Check sheet for the modelled part. Datum: model origin and axes. Units: mm. A direction names the side the tool comes from. Coordinates: 2 decimals unless noted, no trailing zeros. Write each loop counter-clockwise with the first axis right and the second up, starting at its lowest first coordinate (ties: lowest second). Pieces come first, ordered by that corner, then holes. Notation, with made-up numbers: (54.25, -33) - (104.25, -33) arc R12 ccw to (104.25, -11) - close; hole circle Ø5 at (66, 64.5). An arc over 180 degrees is marked (long way). Use one line per item in the form item = value. Start each with the question number.
1. Cross-section at A-A on x = 0. Record the boundary of the cut face in (y, z), then the cut area to 3 significant figures.
2. Tool access check on faces 5 (the face through (-10, 0, 138)), 6 (the face through (10.81, -0.07, 131.45)). Record the directions out of +Z, -Z, +X, -X, +Y, -Y that give a thin tool (end or side, any length) a straight path to the whole face; none if there is none.
3. Draft check along X on faces 1 (the face through (0, 0, 0)), 2 (the face through (-15, 0, 74)), 3 (the face through (-1.08, -0.07, 93.12)), 4 (the face through (15, 0, 74)). Enter one of: +X half, -X half, draft (parallel to the pull), parting line (faces both ways), or undercut.
4. Cross-section at C-C on y = 0. Give the number of separate pieces and of enclosed holes in the cut face, then the cut area to 3 significant figures.
5. Cross-section at D-D on x = 10. Record the boundary of the cut face in (y, z).
6. Cross-section at B-B on z = 45. Record the boundary of the cut face in (x, y), then the cut area to 3 significant figures.
7. Scan lines: line 1 along Z through (x, y) = (10, 2.5); line 2 along X through (y, z) = (-0.5, 133); line 3 along X through (y, z) = (1.5, 97.5). Record each from-to range of solid material in increasing order.
8. Go/stop test with a flat-tipped pin: pin 1 Ø1.5 at (x, y) = (10.5, 0) entering from +Z. Record where the tip stops, or that it passes through.
Autodesk Fusion 360 part; units mm, degrees
sketch "Sketch1" plane through (0, 0, 0) normal (0, 0, 1) x (1, 0, 0)
  line L0 (15, 5) -> (-15, 5)
  line L1 (-15, 5) -> (-15, -5)
  line L2 (-15, -5) -> (15, -5)
  line L3 (15, -5) -> (15, 5)
  line L4 (15, 5) -> (-15, -5) construction
  line L5 (-15, 5) -> (15, -5) construction
  dimension "d1" = 30
  dimension "d2" = 10
extrude "Extrude1" add sketch "Sketch1" along normal blind 150
sketch "Sketch2" plane through (0, -5, 0) normal (0, -1, 0) x (1, 0, 0)
  line L0 (-15, 0) -> (15, 0)
  line L1 (15, 0) -> (15, 150)
  line L2 (15, 150) -> (-15, 150)
  line L3 (-15, 150) -> (-15, 0)
  circle A0 centre (0, 118) radius 1.75
  line L4 (0, 150) -> (0, 118)
  circle A1 centre (-10, 133) radius 1.75
  circle A2 centre (10, 133) radius 1.75
  dimension "d5" = 3.5
  dimension "d6" = 32
  dimension "d7" = 3.5
  dimension "d8" = 3.5
  dimension "d9" = 10
  dimension "d10" = 10
  dimension "d11" = 15
  dimension "d12" = 15
extrude "Extrude2" cut sketch "Sketch2" against normal blind 10 contours A0 | A1 | A2
sketch "Sketch3" plane through (0, 0, 150) normal (0, 0, 1) x (-1, 0, 0)
  line L0 (-15, 5) -> (-15, -5)
  line L1 (-15, -5) -> (15, -5)
  line L2 (15, -5) -> (15, 5)
  line L3 (15, 5) -> (-15, 5)
  circle A0 centre (10, 0) radius 2.05
  circle A1 centre (-10, 0) radius 2.05
  dimension "d15" = 4.1
  dimension "d17" = 10
  dimension "d18" = 10
extrude "Extrude3" cut sketch "Sketch3" against normal blind 12 contours A0 | A1
sketch "Sketch4" plane through (0, -5, 0) normal (0, -1, 0) x (1, 0, 0)
  circle A0 centre (-10, 133) radius 1.75
  circle A1 centre (10, 133) radius 1.75
  circle A2 centre (0, 118) radius 1.75
  line L0 (-15, 0) -> (15, 0)
  line L1 (15, 0) -> (15, 150)
  line L2 (15, 150) -> (-15, 150)
  line L3 (-15, 150) -> (-15, 0)
  line L4 (0, 0) -> (0, 6)
  circle A3 centre (0, 15) radius 1.5
  circle A4 centre (-10, 30) radius 1.5
  circle A5 centre (10, 30) radius 1.5
  circle A6 centre (0, 45) radius 1.5
  dimension "d21" = 3
  dimension "d22" = 15
  dimension "d23" = 3
  dimension "d24" = 10
  dimension "d25" = 30
  dimension "d26" = 3
  dimension "d27" = 45
extrude "Extrude4" cut sketch "Sketch4" against normal blind 10 contours A3 | A4 | A5 | A6
sketch "Sketch5" plane through (0, -5, 0) normal (0, -1, 0) x (1, 0, 0)
  circle A0 centre (0, 45) radius 1.5
  circle A1 centre (10, 30) radius 1.5
  circle A2 centre (-10, 30) radius 1.5
  circle A3 centre (0, 15) radius 1.5
  circle A4 centre (-10, 133) radius 1.75
  circle A5 centre (10, 133) radius 1.75
  circle A6 centre (0, 118) radius 1.75
  line L0 (-15, 0) -> (15, 0)
  line L1 (15, 0) -> (15, 150)
  line L2 (15, 150) -> (-15, 150)
  line L3 (-15, 150) -> (-15, 0)
  circle A7 centre (0, 108) radius 1.75
  dimension "d30" = 3.5
  dimension "d31" = 10
extrude "Extrude5" cut sketch "Sketch5" against normal blind 10 contours A7
sketch "Sketch6" plane through (0, -5, 0) normal (0, -1, 0) x (1, 0, 0)
  circle A0 centre (0, 108) radius 1.75
  circle A1 centre (0, 45) radius 1.5
  circle A2 centre (10, 30) radius 1.5
  circle A3 centre (-10, 30) radius 1.5
  circle A4 centre (0, 15) radius 1.5
  circle A5 centre (-10, 133) radius 1.75
  circle A6 centre (10, 133) radius 1.75
  circle A7 centre (0, 118) radius 1.75
  line L0 (-15, 0) -> (15, 0)
  line L1 (15, 0) -> (15, 150)
  line L2 (15, 150) -> (-15, 150)
  line L3 (-15, 150) -> (-15, 0)
  circle A8 centre (0, 98) radius 5
  dimension "d34" = 10
  dimension "d35" = 10
extrude "Extrude6" cut sketch "Sketch6" against normal blind 10 contours A8
Final values:
q1.outline = (-5, 0) - (5, 0) - (5, 13.5) - (-5, 13.5) - close; (-5, 16.5) - (5, 16.5) - (5, 43.5) - (-5, 43.5) - close; (-5, 46.5) - (5, 46.5) - (5, 93) - (-5, 93) - close; (-5, 103) - (5, 103) - (5, 106.25) - (-5, 106.25) - close; (-5, 109.75) - (5, 109.75) - (5, 116.25) - (-5, 116.25) - close; (-5, 119.75) - (5, 119.75) - (5, 150) - (-5, 150) - close
q1.area = 1,270 mm²
q2.face_5 = +Z
q2.face_6 = +Y, -Y
q3.face_1 = draft
q3.face_2 = -X half
q3.face_3 = undercut
q3.face_4 = +X half
q4.separate_pieces = 1
q4.enclosed_holes = 9
q4.area = 4,260 mm²
q5.outline = (-5, 0) - (5, 0) - (5, 28.5) - (-5, 28.5) - close; (-5, 31.5) - (5, 31.5) - (5, 131.25) - (-5, 131.25) - close; (-5, 134.75) - (5, 134.75) - (5, 150) - (2.05, 150) - (2.05, 138) - (-2.05, 138) - (-2.05, 150) - (-5, 150) - close
q6.outline = (-15, -5) - (-1.5, -5) - (-1.5, 5) - (-15, 5) - close; (1.5, -5) - (15, -5) - (15, 5) - (1.5, 5) - close
q6.area = 270 mm²
q7.line_1 = 0 to 28.5, 31.5 to 131.25, 134.75 to 150
q7.line_2 = -15 to -11.75, -8.25 to 8.25, 11.75 to 15
q7.line_3 = -15 to -4.97, 4.97 to 15
q8.pin_1 = 138
